Drawing for the job (mm, zero at the part's lowest x, y, z). A direction names the side the tool comes from. Give positions to 0.01 mm unless a question says otherwise; leave off trailing zeros. Write each loop counter-clockwise with the first axis right and the second up, starting at its lowest first coordinate (ties: lowest second). Pieces come first, ordered by that corner, then holes.
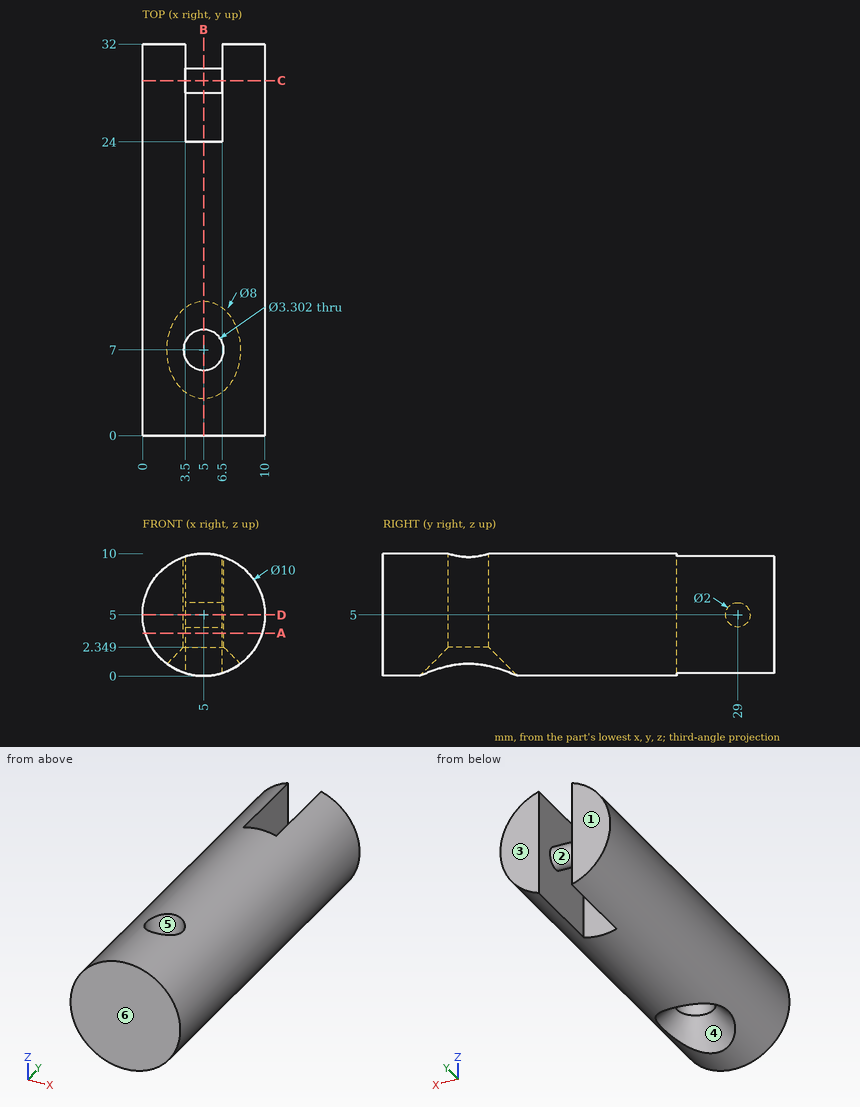
1. Slice it at B-B, the plane x = 5. Write the cut outline in (y, z), and give its area (3 significant figures).
Calculated:
outline: (0, 0) - (3, 0) - (5.35, 2.35) - (5.35, 10) - (0, 10) - close; (8.65, 2.35) - (11, 0) - (24, 0) - (24, 10) - (8.65, 10) - close; circle Ø2 at (29, 5)
area: 205 mm2
2. Pin check, flat tips, straight feed: P1, Ø1, axis at y = 11.5, z = 7.5, coming from the -X side; P2, Ø1, axis at x = 5.5, z = 8, coming from the +Y side; P3, Ø3, axis at x = 8.5, y = 26, coming from the -Z side. Stop position of each tip, or through.
Calculated:
P1: stops at x = 0.42
P2: stops at y = 24
P3: stops at z = 0.42
3. Probe probe 1 along X at (y, z) = (7, 4.75); probe 2 along Y at (x, z) = (3.75, 5); probe 3 along Y at (x, z) = (5.5, 3.25). List the from-to ranges inside material, lowest first.
Calculated:
probe 1: x = 0.01 to 3.35, 6.65 to 9.99
probe 2: y = 0 to 5.92, 8.08 to 24, 28 to 30
probe 3: y = 0 to 5.43, 8.57 to 24
4. Slice it at C-C, the plane y = 29. Write the cut outline in (x, z).
Calculated:
outline: (3.5, 0.23) - (3.5, 4) - (6.5, 4) - (6.5, 0.23) arc R5 ccw to (6.5, 9.77) - (6.5, 6) - (3.5, 6) - (3.5, 9.77) arc R5 ccw to start
5. Slice it at D-D, the plane z = 5. Write the cut outline in (x, y), and give its area (3 significant figures).
Calculated:
outline: (0, 0) - (10, 0) - (10, 32) - (6.5, 32) - (6.5, 30) - (3.5, 30) - (3.5, 32) - (0, 32) - close; hole circle Ø3.3 at (5, 7); hole (3.5, 24) - (6.5, 24) - (6.5, 28) - (3.5, 28) - close
area: 293 mm2
6. Slice it at A-A, the plane z = 3.5. Write the cut outline in (x, y), and give its area (3 significant figures).
Calculated:
outline: (0.23, 0) - (9.77, 0) - (9.77, 32) - (6.5, 32) - (6.5, 24) - (3.5, 24) - (3.5, 32) - (0.23, 32) - close; hole circle Ø3.3 at (5, 7)
area: 273 mm2
7. Which spindle directions (+Z, -Z, +X, -X, +Y, -Y) get a long thin tool onto all of the face, cutting with end or side? Do the marked faces 1 and 2. Say none if no direction does.
Calculated:
face 1: +Z, -Z, +X, -X, +Y
face 2: none
8. Pull direction Y, two halves, no side cores. Call the marked faces 3, 4, 5 and 6: +Y half, -Y half, draft (parallel to the pull), parting line (faces both ways), or undercut.
Calculated:
face 3: +Y half
face 4: undercut
face 5: undercut
face 6: -Y half
